Source: three-view drawing plus pictorial views. Frame: mm from the lowest corner of the part. A direction names the side the tool comes from. Coordinates: 2 decimals unless noted, no trailing zeros. Loops run counter-clockwise (first coordinate to the right, second up) from the corner with the lowest first, then second, coordinate; pieces in that order, holes last. Notation, with made-up numbers: M 40.5,39 L 65.5,39 A35 cw 65.5,74 Z; hole C -13.5,50 d7. An arc over 180 degrees is marked long. Use a Markdown table: item, result. Add a question column.
1. Set-up query: the marked faces 1, 2 and 3. Return all of +Z, -Z, +X, -X, +Y, -Y with unobstructed straight access to the full face (end or side cutting, diameter ignored); none if empty.
2. Section A-A on y = 1.85. Output: boundary loops of the cut face in (x, z), then the cut area to 3 significant figures.
3. Section C-C on y = 2.4. Output: boundary loops of the cut face in (x, z).
4. Section B-B on x = 8. Output: boundary loops of the cut face in (y, z).
5. Line query: L1, parallel to Z at x = 1, y = 2.45; L2, parallel to X at y = 0.4, z = 5.75. Output: solid intervals per line, ascending. Write a range as [from, to].
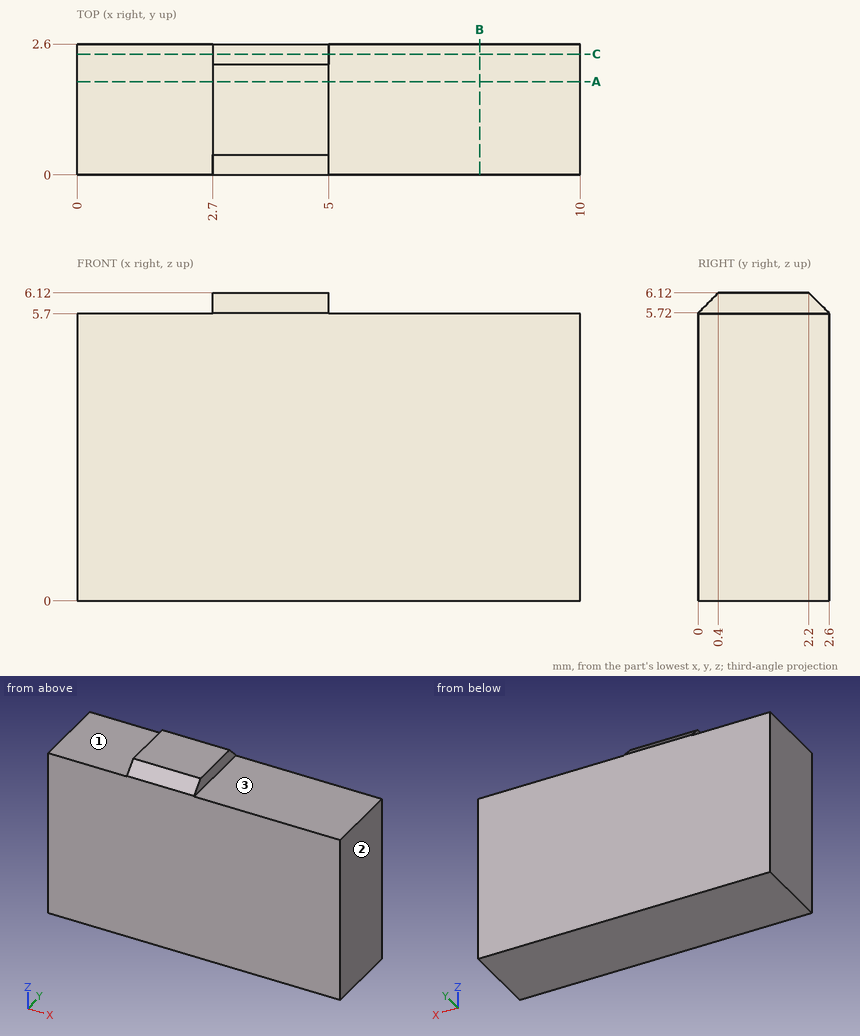
Answers below:
| question | item | result |
|---|---|---|
| 1 | face 1 | +Z, -X, +Y, -Y |
| 1 | face 2 | +Z, -Z, +X, +Y, -Y |
| 1 | face 3 | +Z, +X, +Y, -Y |
| 2 | outline | M 0,0 L 10,0 L 10,5.7 L 5,5.7 L 5,6.12 L 2.7,6.12 L 2.7,5.7 L 0,5.7 Z |
| 2 | area | 58.0 mm² |
| 3 | outline | M 0,0 L 10,0 L 10,5.7 L 5,5.7 L 5,5.92 L 2.7,5.92 L 2.7,5.7 L 0,5.7 Z |
| 4 | outline | M 0,0 L 2.6,0 L 2.6,5.7 L 0,5.7 Z |
| 5 | L1 | z = [0, 5.7] |
| 5 | L2 | x = [2.7, 5] |
